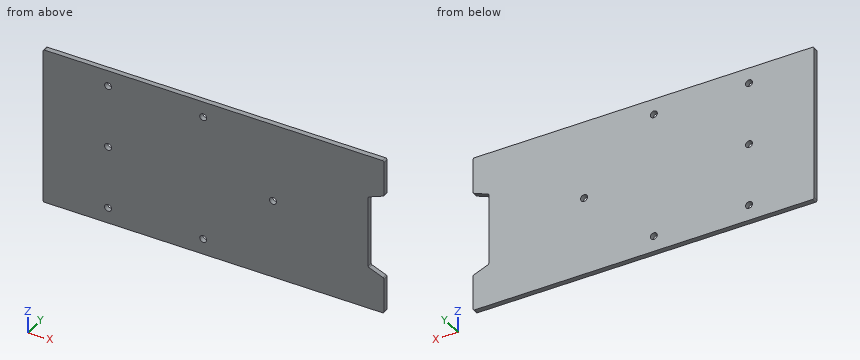
from build123d import *

# Parameters (mm, degrees)
BOSS_EXTRUDE1_DEPTH = 1.6
SKETCH2_R           = 1.1
CUT_EXTRUDE1_DEPTH  = 119.569852829


with BuildPart() as part:
    # Sketch1 → Boss-Extrude1 (new body)
    with BuildSketch(Plane(origin=(0, 0, 0), x_dir=(1, 0, 0), z_dir=(0, 1, 0))):
        with BuildLine():
            Line((102.5, 50), (106.992600234, 50))
            ThreePointArc((106.992600234, 50), (107.351386049, 49.851386049), (107.5, 49.492600234))
            Line((107.5, 49.492600234), (107.5, 38.843526366))
            ThreePointArc((107.5, 38.843526366), (107.412761353, 38.55906344), (107.181043776, 38.372417511))
            Line((107.181043776, 38.372417511), (102.818956224, 36.627582489))
            ThreePointArc((102.818956224, 36.627582489), (102.587238647, 36.44093656), (102.5, 36.156473634))
            Line((102.5, 36.156473634), (102.5, 13.843526366))
            ThreePointArc((102.5, 13.843526366), (102.587238647, 13.55906344), (102.818956224, 13.372417511))
            Line((102.818956224, 13.372417511), (107.181043776, 11.627582489))
            ThreePointArc((107.181043776, 11.627582489), (107.412761353, 11.44093656), (107.5, 11.156473634))
            Line((107.5, 11.156473634), (107.5, 0.507399766))
            ThreePointArc((107.5, 0.507399766), (107.351386049, 0.148613951), (106.992600234, 0))
            Line((106.992600234, 0), (102.5, 0))
            Line((102.5, 0), (0.507399766, 0))
            ThreePointArc((0.507399766, 0), (0.148613951, 0.148613951), (0, 0.507399766))
            Line((0, 0.507399766), (0, 49.492600234))
            ThreePointArc((0, 49.492600234), (0.148613951, 49.851386049), (0.507399766, 50))
            Line((0.507399766, 50), (102.5, 50))
        make_face()
    extrude(amount=BOSS_EXTRUDE1_DEPTH)

    # Sketch2 → Cut-Extrude1 (cut, through all)
    with BuildSketch(Plane(origin=(0, 1.6, 0), x_dir=(1, 0, 0), z_dir=(0, 1, 0))):
        with Locations(Location((20.5, 5, 0), (0, 0, 270))):
            Circle(SKETCH2_R)
        with Locations(Location((20.5, 25, 0), (0, 0, 270))):
            Circle(SKETCH2_R)
        with Locations(Location((20.5, 45, 0), (0, 0, 270))):
            Circle(SKETCH2_R)
        with Locations(Location((50.5, 45, 0), (0, 0, 270))):
            Circle(SKETCH2_R)
        with Locations(Location((50.5, 5, 0), (0, 0, 270))):
            Circle(SKETCH2_R)
        with Locations(Location((72.5, 25, 0), (0, 0, 270))):
            Circle(SKETCH2_R)
    extrude(amount=-CUT_EXTRUDE1_DEPTH, mode=Mode.SUBTRACT)


solid = part.part
Can you work these out from the model? Positions are in its coordinate system, mm. Round coordinates to 2 decimals unless told otherwise and drop trailing zeros. Write each loop counter-clockwise with the first axis right and the second up, starting at its lowest first coordinate (ties: lowest second). Pieces come first, ordered by that corner, then holes. Notation, with made-up numbers: (15, -20) -> (38, -20) arc R18 ccw to (38, 12) -> close; hole circle Ø1 at (19, -14.5). An arc over 180 degrees is marked (long way). One line per question, with ' | ' between items. Start each with the question number.
1) Suppose I cut it at C-C on y = 0.85. Write out the boundary of the cut face in (x, z).
2) Suppose I cut it at D-D on x = 20.5. Write out the boundary of the cut face in (y, z), then the cut area to 3 significant figures.
3) I need wall thicknesses on line 1 (X direction, y = 1.25, z = -5); line 2 (X direction, y = 1.35, z = -25); line 3 (Z direction, x = 72.5, y = 0.6). Which ranges of each line are inside material? Lowest first, please. Write a range as [from, to].
4) Suppose I cut it at A-A on x = 72.5. Write out the boundary of the cut face in (y, z), then the cut area to 3 significant figures.
5) Suppose I cut it at B-B on z = -45. Write out the boundary of the cut face in (x, y).
Return value:
1) outline: (0, -49.49) arc R0.51 ccw to (0.51, -50) -> (106.99, -50) arc R0.51 ccw to (107.5, -49.49) -> (107.5, -38.84) arc R0.51 ccw to (107.18, -38.37) -> (102.82, -36.63) arc R0.51 cw to (102.5, -36.16) -> (102.5, -13.84) arc R0.51 cw to (102.82, -13.37) -> (107.18, -11.63) arc R0.51 ccw to (107.5, -11.16) -> (107.5, -0.51) arc R0.51 ccw to (106.99, 0) -> (0.51, 0) arc R0.51 ccw to (0, -0.51) -> close; hole circle Ø2.2 at (20.5, -45); hole circle Ø2.2 at (20.5, -25); hole circle Ø2.2 at (20.5, -5); hole circle Ø2.2 at (50.5, -45); hole circle Ø2.2 at (50.5, -5); hole circle Ø2.2 at (72.5, -25)
2) outline: (0, -50) -> (1.6, -50) -> (1.6, -46.1) -> (0, -46.1) -> close; (0, -43.9) -> (1.6, -43.9) -> (1.6, -26.1) -> (0, -26.1) -> close; (0, -23.9) -> (1.6, -23.9) -> (1.6, -6.1) -> (0, -6.1) -> close; (0, -3.9) -> (1.6, -3.9) -> (1.6, 0) -> (0, 0) -> close | area: 69.4 mm2
3) line 1: x = [0, 19.4], [21.6, 49.4], [51.6, 107.5] | line 2: x = [0, 19.4], [21.6, 71.4], [73.6, 102.5] | line 3: z = [-50, -26.1], [-23.9, 0]
4) outline: (0, -50) -> (1.6, -50) -> (1.6, -26.1) -> (0, -26.1) -> close; (0, -23.9) -> (1.6, -23.9) -> (1.6, 0) -> (0, 0) -> close | area: 76.5 mm2
5) outline: (0, 0) -> (19.4, 0) -> (19.4, 1.6) -> (0, 1.6) -> close; (21.6, 0) -> (49.4, 0) -> (49.4, 1.6) -> (21.6, 1.6) -> close; (51.6, 0) -> (107.5, 0) -> (107.5, 1.6) -> (51.6, 1.6) -> close
